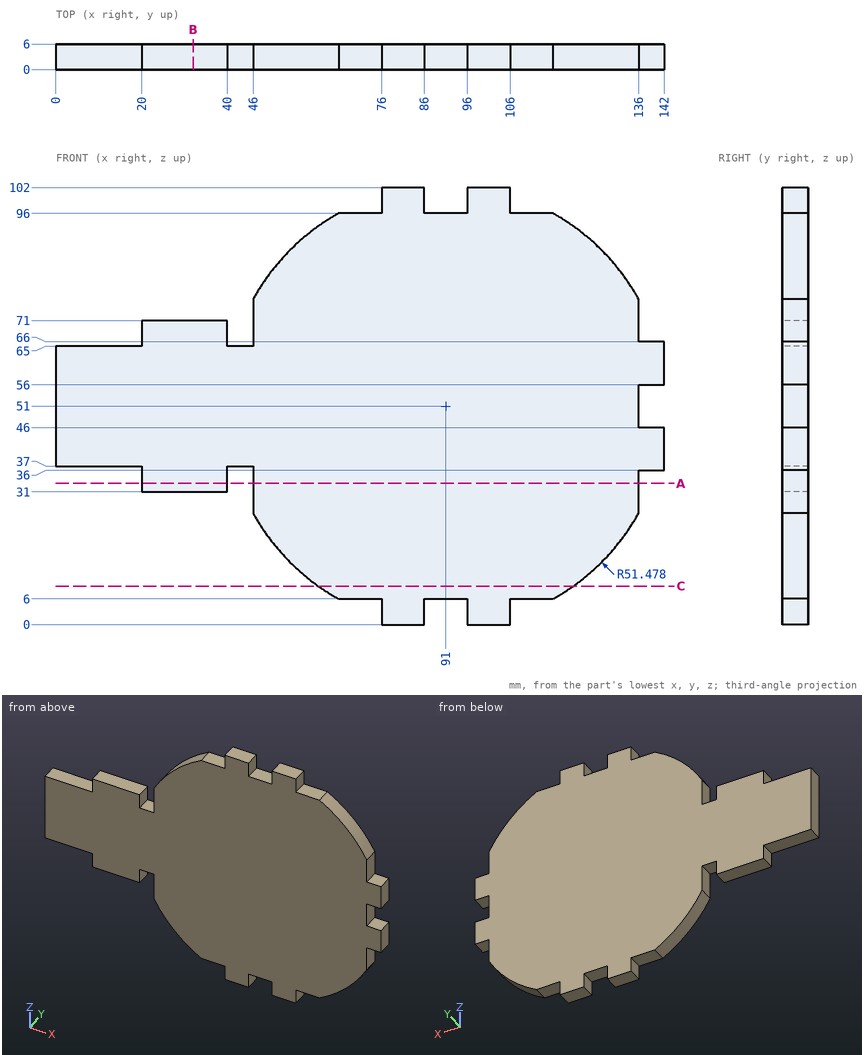
Input: dimensioned drawing with shaded views. Units: mm. Origin: part minimum x, y, z. Give positions to 0.01 mm unless a question says otherwise; leave off trailing zeros. Write each loop counter-clockwise with the first axis right and the second up, starting at its lowest first coordinate (ties: lowest second). Pieces come first, ordered by that corner, then holes. Notation, with made-up numbers: M -39.75,-28.75 L 2.25,-28.75 A33 cw 2.25,6.25 Z; hole C 33.25,39.25 d11. An arc over 180 degrees is marked long. Write item = value, one per line. Start each with the question number.
1) Cut plane C-C on z = 9. Return the cut outline in (x, y).
2) Cut plane B-B on x = 32. Return the cut outline in (y, z).
3) First-contact query: pin 1 Ø3 at (y, z) = (4, 33) entering from +X; pin 2 Ø3 at (x, y) = (29.5, 2) entering from -Z; pin 3 Ø3 at (y, z) = (2.5, 2.5) entering from +X. Flat tips, straight axial feed; report the tip coordinate or a pass-through.
4) Cut plane A-A on z = 33. Return the cut outline in (x, y).
5) Material intervals for line 1 along X through (y, z) = (1.1, 4); line 2 along X through (y, z) = (1.15, 34); line 3 along X through (y, z) = (4.2, 29.5), sorted ascending. Write a range as [from, to].
Solved:
q1.outline = M 61.23,0 L 120.77,0 L 120.77,6 L 61.23,6 Z
q2.outline = M 0,31 L 6,31 L 6,71 L 0,71 Z
q3.pin_1 = 136
q3.pin_2 = 31
q3.pin_3 = 106
q4.outline = M 20,0 L 40,0 L 40,6 L 20,6 Z; M 46,0 L 136,0 L 136,6 L 46,6 Z
q5.line_1 = [76, 86], [96, 106]
q5.line_2 = [20, 40], [46, 136]
q5.line_3 = [46, 136]
